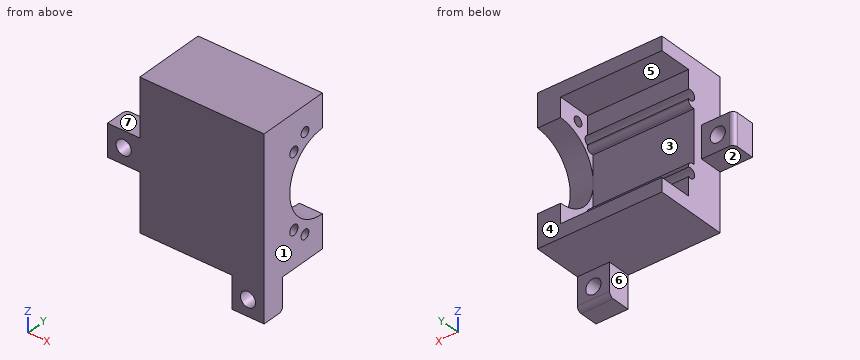
from build123d import *

# Parameters (mm, degrees)
BOSS_EXTRUDE1_DEPTH = 11
SKETCH3_W           = 22
SKETCH3_H           = 3
BOSS_EXTRUDE2_DEPTH = 15.7
BOSS_EXTRUDE3_DEPTH = 5
SKETCH5_R           = 1.035
SKETCH5_R_2         = 1.1
CUT_EXTRUDE1_DEPTH  = 36.096650541
SKETCH6_W           = 7
SKETCH6_H           = 7
BOSS_EXTRUDE4_DEPTH = 5
SKETCH7_R           = 1.65
CUT_EXTRUDE2_DEPTH  = 32.1110829
FILLET1_R           = 1


with BuildPart() as part:
    # Sketch1 → Boss-Extrude1 (new, symmetric)
    with BuildSketch(Plane(origin=(0, 0, 0), x_dir=(0, 0, -1), z_dir=(1, 0, 0))):
        Polygon((-13.0089, 0), (13.0089, 0), (13.0089, 8.5), (5.7589, 8.5), (5.7589, 7), (-5.7589, 7), (-5.7589, 8.5), (-13.0089, 8.5), align=None)
    extrude(amount=BOSS_EXTRUDE1_DEPTH, both=True)

    # Sketch3 → Boss-Extrude2 (add)
    with BuildSketch(Plane.XZ):
        with Locations((0, -14.5089)):
            Rectangle(SKETCH3_W, SKETCH3_H)
        with Locations((0, 14.5089)):
            Rectangle(SKETCH3_W, SKETCH3_H)
    extrude(amount=-BOSS_EXTRUDE2_DEPTH)

    # Sketch4 → Boss-Extrude3 (add)
    with BuildSketch(Plane(origin=(11, 0, 0), x_dir=(0, 0, -1), z_dir=(1, 0, 0))):
        with BuildLine():
            Line((-8.8, 15.7), (-16.0089, 15.7))
            Line((-16.0089, 15.7), (-16.0089, 0))
            Line((-16.0089, 0), (16.0089, 0))
            Line((16.0089, 0), (16.0089, 15.7))
            Line((16.0089, 15.7), (8.8, 15.7))
            ThreePointArc((8.8, 15.7), (0, 6.9), (-8.8, 15.7))
        make_face()
    extrude(amount=BOSS_EXTRUDE3_DEPTH)

    # Sketch5 → Cut-Extrude1 (cut, through all)
    with BuildSketch(Plane(origin=(16, 0, 0), x_dir=(0, 0, -1), z_dir=(1, 0, 0))):
        with Locations((-10.5, 11)):
            Circle(SKETCH5_R)
        with Locations((10.5, 11)):
            Circle(SKETCH5_R)
        with Locations((-8.0089, 8)):
            Circle(SKETCH5_R_2)
        with Locations(Location((8.0089, 8, 0), (0, 0, 27.035691789))):
            Circle(SKETCH5_R_2)
    extrude(amount=-CUT_EXTRUDE1_DEPTH, mode=Mode.SUBTRACT)

    # Sketch6 → Boss-Extrude4 (add)
    with BuildSketch(Plane.XZ):
        with Locations((12.5, -19.5089)):
            Rectangle(SKETCH6_W, SKETCH6_H)
        with Locations((-14.5, 0)):
            Rectangle(SKETCH6_W, SKETCH6_H)
    extrude(amount=-BOSS_EXTRUDE4_DEPTH)

    # Sketch7 → Cut-Extrude2 (cut, through all)
    with BuildSketch(Plane(origin=(0, 5, 0), x_dir=(1, 0, 0), z_dir=(0, 1, 0))):
        with Locations(Location((-14.5, 0, 0), (0, 0, 270))):
            Circle(SKETCH7_R)
        with Locations(Location((12.5, 19.5089, 0), (0, 0, 270))):
            Circle(SKETCH7_R)
    extrude(amount=-CUT_EXTRUDE2_DEPTH, mode=Mode.SUBTRACT)

    # Fillet1
    fillet1_edges = [part.edges().sort_by_distance(p)[0] for p in [
        (-18, 5, 0),
        (12.5, 5, -23.0089),
        (0, 8.5, 5.7589),
        (0, 8.5, -5.7589),
    ]]
    fillet(fillet1_edges, radius=FILLET1_R)


solid = part.part
Design review of the part built by this model. Coordinates are the model's own, in mm. Face numbers are marked on the shaded views. A direction names the side the tool comes from. Give positions to 0.01 mm unless a question says otherwise; leave off trailing zeros. Write each loop counter-clockwise with the first axis right and the second up, starting at its lowest first coordinate (ties: lowest second). Pieces come first, ordered by that corner, then holes. Notation, with made-up numbers: M 86,32 L 145,32 A5 cw 145,38 Z; hole C 27,55 d6. An arc over 180 degrees is marked long. Return JSON: item names as keys, results as strings. Group by question number.
Item 1: Take a section at D-D (x = -14.5). Give the boundary of the cut face in (y, z), plus the area to 3 significant figures.
Item 2: Take a section at A-A (x = 13). Give the boundary of the cut face in (y, z) (3 decimals), plus the area to 3 significant figures.
Item 3: Take a section at B-B (z = 10.5). Give the boundary of the cut face in (x, y) (3 decimals), plus the area to 3 significant figures.
Item 4: The part is to be moulded in two halves that separate along Z. For the marked faces 1, 2 and 3, say which applies: pulls with the +Z half, pulls with the -Z half, needs draft (parallel to the pull), parting line crosses it, or undercut.
Item 5: Take a section at C-C (y = 8). Give the boundary of the cut face in (x, z), plus the area to 3 significant figures.
Item 6: Tool access review of the marked faces 4, 5, 6 and 7: name each direction out of +Z, -Z, +X, -X, +Y, -Y from which nothing blocks a thin tool from reaching the whole face with its end or side.
Item 7: Wall thickness on line 1 along Y through (x, z) = (12, 8); line 2 along Z through (x, y) = (8.75, 8); line 3 along X through (y, z) = (1.5, -4.5): over which ranges is each line inside the solid? List them lowest first.
Item 8: Clearance check with flat-ended pins moving along their axes: pin 1 Ø2 at (x, y) = (-10, 8.5) entering from -Z; pin 2 Ø2 at (x, z) = (5, -10) entering from +Y; pin 3 Ø2.5 at (x, y) = (-16, 3) entering from +Z. State where each tip first meets the part, or that it passes through.
Return value:
{
 "1": {"outline": "M 0,-3.5 L 5,-3.5 L 5,-1.65 L 0,-1.65 Z; M 0,1.65 L 5,1.65 L 5,3.5 L 0,3.5 Z", "area": "18.5 mm2"},
 "2": {"outline": "M 0,-23.009 L 4,-23.009 A1 ccw 5,-22.009 L 5,-21.081 L 0,-21.081 Z; M 0,-17.936 L 5,-17.936 L 5,-16.009 L 15.7,-16.009 L 15.7,-8.8 A8.8 cw 15.7,8.8 L 15.7,16.009 L 0,16.009 Z; hole C 8,-8.009 d2.2; hole C 8,8.009 d2.2; hole C 11,-10.5 d2.07; hole C 11,10.5 d2.07", "area": "386 mm2"},
 "3": {"outline": "M -11,0 L 16,0 L 16,9.965 L 11,9.965 L 11,8.5 L -11,8.5 Z; M 11,12.035 L 16,12.035 L 16,15.7 L 11,15.7 Z", "area": "255 mm2"},
 "4": {"face 1": "needs draft", "face 2": "pulls with the -Z half", "face 3": "undercut"},
 "5": {"outline": "M -11,-16.01 L 16,-16.01 L 16,-9.11 L -11,-9.11 Z; M -11,-6.91 L 16,-6.91 L 16,-4.26 L 11,-4.26 L 11,-5.89 L -11,-5.89 Z; M -11,5.89 L 11,5.89 L 11,4.26 L 16,4.26 L 16,6.91 L -11,6.91 Z; M -11,9.11 L 16,9.11 L 16,16.01 L -11,16.01 Z", "area": "444 mm2"},
 "6": {"face 4": "+Z, -Z, +X, -X, +Y", "face 5": "-X, +Y", "face 6": "-Z, -X, +Y, -Y", "face 7": "+Z, -X, +Y, -Y"},
 "7": {"line 1": "y = 0 to 6.9, 9.1 to 12.03", "line 2": "z = -16.01 to -9.11, -6.91 to -5.89, 5.89 to 6.91, 9.11 to 16.01", "line 3": "x = -11 to 16"},
 "8": {"pin 1": "stops at z = -16.01", "pin 2": "stops at y = 8.5", "pin 3": "stops at z = 3.5"}
}
